The listing builds one solid part. Answer for the finished solid, in the listing's coordinates (mm). A direction names the side the tool comes from. Give positions to 0.01 mm unless a question says otherwise; leave off trailing zeros. Order: outer loops, then holes, each group sorted by start corner. A loop starts at its lowest first (then second) coordinate and runs counter-clockwise, first axis right, second up.
```python
from build123d import *

# Parameters (mm, degrees)
SKETCH1_R           = 19.75
SKETCH1_R_2         = 4.2
SKETCH1_R_3         = 1.25
BOSS_EXTRUDE1_DEPTH = 3.175
SKETCH3_R           = 19.95
SKETCH3_R_2         = 11.95
BOSS_EXTRUDE2_DEPTH = 13.325
SKETCH4_R           = 2
CUT_EXTRUDE1_DEPTH  = 42.12243913
CIRPATTERN1_COUNT   = 4
SKETCH5_R           = 24.6
SKETCH5_R_2         = 19.75
BOSS_EXTRUDE3_DEPTH = 8
CHAMFER1_SIZE       = 0.5
FILLET1_R           = 1.5


with BuildPart() as part:
    # Sketch1 → Boss-Extrude1 (new body)
    with BuildSketch(Plane.XY):
        with Locations((0, 12)):
            Circle(SKETCH1_R)
        with Locations((0, 12)):
            Circle(SKETCH1_R_2, mode=Mode.SUBTRACT)
        with Locations((5.656854249, 17.656854249)):
            Circle(SKETCH1_R_3, mode=Mode.SUBTRACT)
        with Locations((8, 12)):
            Circle(SKETCH1_R_3, mode=Mode.SUBTRACT)
        with Locations((5.656854249, 6.343145751)):
            Circle(SKETCH1_R_3, mode=Mode.SUBTRACT)
        with Locations((0, 4)):
            Circle(SKETCH1_R_3, mode=Mode.SUBTRACT)
        with Locations((-5.656854249, 6.343145751)):
            Circle(SKETCH1_R_3, mode=Mode.SUBTRACT)
        with Locations((-8, 12)):
            Circle(SKETCH1_R_3, mode=Mode.SUBTRACT)
        with Locations((-5.656854249, 17.656854249)):
            Circle(SKETCH1_R_3, mode=Mode.SUBTRACT)
        with Locations((0, 20)):
            Circle(SKETCH1_R_3, mode=Mode.SUBTRACT)
    extrude(amount=BOSS_EXTRUDE1_DEPTH)

    # Sketch3 → Boss-Extrude2 (add)
    with BuildSketch(Plane.XY.offset(3.175)):
        with Locations((0, 12)):
            Circle(SKETCH3_R)
        with Locations((0, 12)):
            Circle(SKETCH3_R_2, mode=Mode.SUBTRACT)
    extrude(amount=BOSS_EXTRUDE2_DEPTH)

    # Sketch4 → Cut-Extrude1 (cut, through all)
    with BuildSketch(Plane.XY.offset(16.5)):
        with Locations((-15.95, 12)):
            Circle(SKETCH4_R)
    cut_extrude1 = extrude(amount=-CUT_EXTRUDE1_DEPTH, mode=Mode.SUBTRACT)

    # CirPattern1: Cut-Extrude1 ×4 about axis
    cirpattern1_axis = Axis((0, 12, 0), (0, 0, 1))
    for i in range(1, CIRPATTERN1_COUNT):
        add(cut_extrude1.rotate(cirpattern1_axis, i * 360 / CIRPATTERN1_COUNT), mode=Mode.SUBTRACT)

    # Sketch5 → Boss-Extrude3 (add)
    with BuildSketch(Plane(origin=(0, 0, 0), x_dir=(-1, 0, 0), z_dir=(0, 0, -1))):
        with Locations((0, 12)):
            Circle(SKETCH5_R)
        with Locations((0, 12)):
            Circle(SKETCH5_R_2, mode=Mode.SUBTRACT)
    extrude(amount=-BOSS_EXTRUDE3_DEPTH)

    # Chamfer1
    chamfer1_edges = [part.edges().sort_by_distance(p)[0] for p in [
        (-17.95, 12, 16.5),
        (0, -5.95, 16.5),
        (17.95, 12, 16.5),
        (0, 29.95, 16.5),
    ]]
    chamfer(chamfer1_edges, length=CHAMFER1_SIZE)

    # Fillet1
    fillet1_edges = [part.edges().sort_by_distance(p)[0] for p in [
        (-11.95, 12, 3.175),
    ]]
    fillet(fillet1_edges, radius=FILLET1_R)


solid = part.part
```
1) Find section B-B (x = 15.95). Write down the section's boundary in (y, z), then the cut area to 3 significant figures.
Geometry says:
outline: (-6.73, 0) - (10, 0) - (10, 16) - (9.5, 16.5) - (0.02, 16.5) - (0.02, 8) - (-6.73, 8) - close; (14, 0) - (30.73, 0) - (30.73, 8) - (23.98, 8) - (23.98, 16.5) - (14.5, 16.5) - (14, 16) - close
area: 437 mm2
2) Given P1, Ø3, axis at x = -12, z = 10.5, coming from the +Y side; P2, Ø8, axis at x = -19.5, z = 5, coming from the -Y side; P3, Ø10.5, axis at x = 3.5, y = 14, coming from the +Z side (3 decimals), each flat-ended and moving along its own axis, determine where each tip first touches the part or whether it passes through.
Geometry says:
P1: stops at y = 28.96
P2: stops at y = -7.1
P3: stops at z = 3.175
3) Find section C-C (z = 13.5). Write down the section's boundary in (x, y).
Geometry says:
outline: circle Ø39.9 at (0, 12); hole circle Ø4 at (-15.95, 12); hole circle Ø23.9 at (0, 12); hole circle Ø4 at (0, -3.95); hole circle Ø4 at (0, 27.95); hole circle Ø4 at (15.95, 12)
4) Find section D-D (z = 2.25). Count the separate pieces of the cut face and the enclosed holes in it, then the cut area to 3 significant figures.
Geometry says:
separate pieces: 1
enclosed holes: 13
area: 1,760 mm2
5) Find section A-A (y = 27.95). Write down the section's boundary in (x, z).
Geometry says:
outline: (-18.73, 0) - (-2, 0) - (-2, 16) - (-2.5, 16.5) - (-11.98, 16.5) - (-11.98, 8) - (-18.73, 8) - close; (2, 0) - (18.73, 0) - (18.73, 8) - (11.98, 8) - (11.98, 16.5) - (2.5, 16.5) - (2, 16) - close
6) A tool of negligible diameter and unlimited length cuts with its end or side. For faces 4 (the cylindrical face through (-0.27, 18.78, 1.57)), 5 (the flat face through (0.1, 32.2, 8)), from which of +Z, -Z, +X, -X, +Y, -Y can it reach the whole face along a straight path? Write none if from no direction.
Geometry says:
face 4: +Z, -Z
face 5: +Z
7) Straight lines are drawn through the part: probe 1 along Y at (x, z) = (1.5, 14); probe 2 along Z at (x, y) = (-4, 6) (3 decimals); probe 3 along Z at (x, y) = (-15.5, -4). For each, find the intervals that lie inside material, in ascending order.
Geometry says:
probe 1: y = -7.89 to -5.27, -2.63 to 0.14, 23.86 to 26.63, 29.27 to 31.89
probe 2: z = 0 to 3.175
probe 3: z = 0 to 8
8) For a pull along X with two mould halves and no side action, classify faces 1 (the cylindrical face through (-22.724, 2.578, 3.944)), 2 (the cylindrical face through (-0.547, 16.164, 1.565)), 3 (the flat face through (9, 3, 16.5)) as +X half, -X half, draft (parallel to the pull), parting line (faces both ways), or undercut.
Geometry says:
face 1: parting line
face 2: undercut
face 3: draft
